Source: three-view drawing plus pictorial views. Frame: mm from the lowest corner of the part. A direction names the side the tool comes from. Give positions to 0.01 mm unless a question says otherwise; leave off trailing zeros. Order: outer loops, then holes, each group sorted by start corner. A loop starts at its lowest first (then second) coordinate and runs counter-clockwise, first axis right, second up.
1) Access query for the marked faces 1 and 2. Directions: +Z, -Z, +X, -X, +Y, -Y. A direction counts if a zero-diameter tool reaches every point of the face in a straight line with its end or side. Return the directions, or none.
2) Draft query along X for the marked faces 3, 4 and 5. Return one class per face: released by +X, released by -X, zero draft, split by the parting line, or undercut.
3) Section A-A, the plane z = 5.25. Return loops of the section in (x, y).
4) Section C-C, the plane y = 25.5. Return loops of the section in (x, z), plus the area to 3 significant figures.
5) Section B-B, the plane y = 20.5. Return loops of the section in (x, z), plus the area to 3 significant figures.
6) Material intervals for line 1 (X direction, y = 29, z = 14); line 2 (X direction, y = 20.5, z = 11); line 3 (Y direction, x = 29, z = 4), sorted ascending.
7) Section D-D, the plane x = 31.5. Return loops of the section in (y, z), plus the area to 3 significant figures.
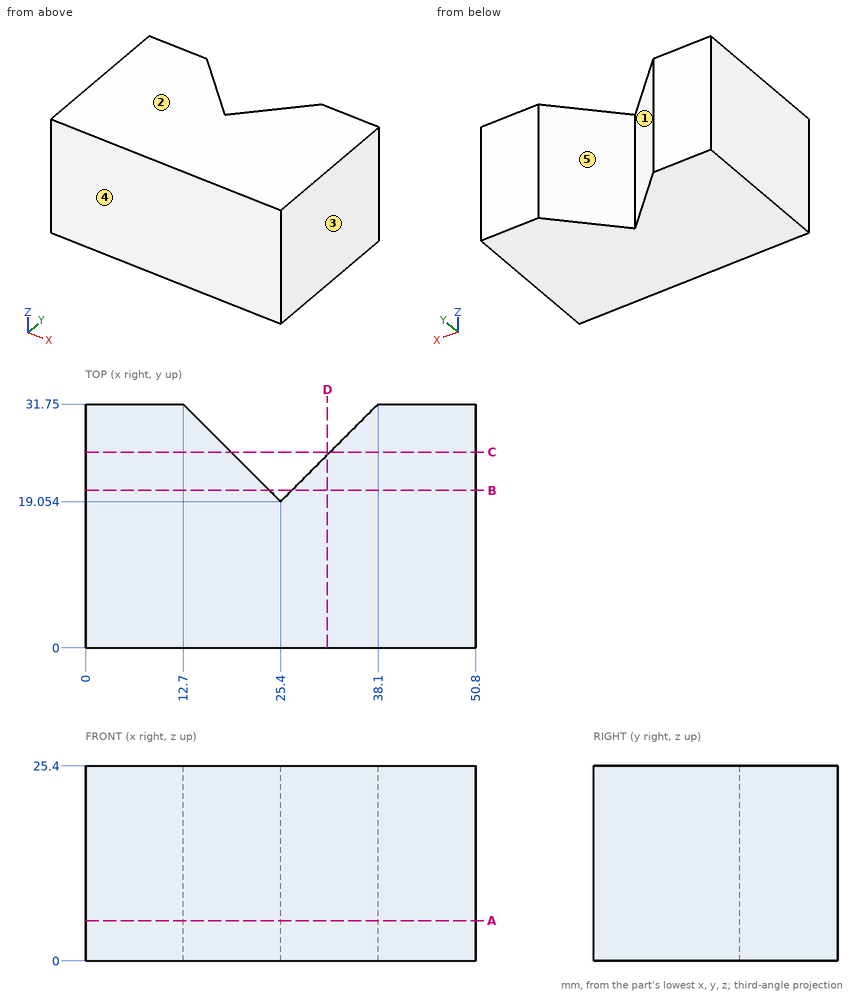
From the geometry:
1. face 1: +Z, -Z, +Y
1. face 2: +Z, +X, -X, +Y, -Y
2. face 3: released by +X
2. face 4: zero draft
2. face 5: undercut
3. outline: (0, 0) - (50.8, 0) - (50.8, 31.75) - (38.1, 31.75) - (25.4, 19.05) - (12.7, 31.75) - (0, 31.75) - close
4. outline: (0, 0) - (18.95, 0) - (18.95, 25.4) - (0, 25.4) - close; (31.85, 0) - (50.8, 0) - (50.8, 25.4) - (31.85, 25.4) - close
4. area: 963 mm2
5. outline: (0, 0) - (23.95, 0) - (23.95, 25.4) - (0, 25.4) - close; (26.85, 0) - (50.8, 0) - (50.8, 25.4) - (26.85, 25.4) - close
5. area: 1,220 mm2
6. line 1: x = 0 to 15.45, 35.35 to 50.8
6. line 2: x = 0 to 23.95, 26.85 to 50.8
6. line 3: y = 0 to 22.65
7. outline: (0, 0) - (25.15, 0) - (25.15, 25.4) - (0, 25.4) - close
7. area: 639 mm2
